Could you check a few things on this model? Use its own coordinates, in mm. Face numbers are marked on the shaded views. Coordinates: 2 decimals unless noted, no trailing zeros. Order: outer loops, then holes, each group sorted by start corner. A loop starts at its lowest first (then second) coordinate and runs counter-clockwise, first axis right, second up. Notation, with made-up numbers: (9.5, 81.25) - (18.5, 81.25) arc R19 cw to (18.5, 117.25) - close; hole circle Ø9 at (30, -0.5). An arc over 180 degrees is marked (long way). One line per item, written item: value.
from build123d import *

# Parameters (mm, degrees)
EXTRUDE_1_DEPTH     = 1.56
SKETCH_3_W          = 59.16
SKETCH_3_H          = 29.5
EXTRUDE_2_DEPTH     = 1
SKETCH_8_W          = 51
SKETCH_8_H          = 5
EXTRUDE_6_DEPTH     = 3.68
SKETCH_9_W          = 49.12
SKETCH_9_H          = 24.52
CUT_EXTRUDE_1_DEPTH = 0.1


with BuildPart() as part:
    # 草图1 → 凸台-拉伸1 (new body)
    with BuildSketch(Plane(origin=(0, 0, 0), x_dir=(1, 0, 0), z_dir=(0, 1, 0))):
        with BuildLine():
            Line((-29.5, 15.375), (29.5, 15.375))
            ThreePointArc((29.5, 15.375), (31.621320344, 14.496320344), (32.5, 12.375))
            Line((32.5, 12.375), (32.5, -12.375))
            ThreePointArc((32.5, -12.375), (31.621320344, -14.496320344), (29.5, -15.375))
            Line((29.5, -15.375), (-29.5, -15.375))
            ThreePointArc((-29.5, -15.375), (-31.621320344, -14.496320344), (-32.5, -12.375))
            Line((-32.5, -12.375), (-32.5, 12.375))
            ThreePointArc((-32.5, 12.375), (-31.621320344, 14.496320344), (-29.5, 15.375))
        make_face()
    extrude(amount=EXTRUDE_1_DEPTH)

    # 草图3 → 凸台-拉伸2 (add)
    with BuildSketch(Plane(origin=(0, 1.56, 0), x_dir=(1, 0, 0), z_dir=(0, 1, 0))):
        with Locations((0.06, -0.125)):
            Rectangle(SKETCH_3_W, SKETCH_3_H)
    extrude(amount=EXTRUDE_2_DEPTH)

    # 草图8 → 凸台-拉伸6 (add)
    with BuildSketch(Plane.XZ):
        with Locations((-0.2, -11.235)):
            Rectangle(SKETCH_8_W, SKETCH_8_H)
    extrude(amount=EXTRUDE_6_DEPTH)

    # 草图9 → 切除-拉伸1 (cut)
    with BuildSketch(Plane(origin=(0, 2.56, 0), x_dir=(1, 0, 0), z_dir=(0, 1, 0))):
        with Locations((2.45, -0.235)):
            Rectangle(SKETCH_9_W, SKETCH_9_H)
    extrude(amount=-CUT_EXTRUDE_1_DEPTH, mode=Mode.SUBTRACT)


solid = part.part
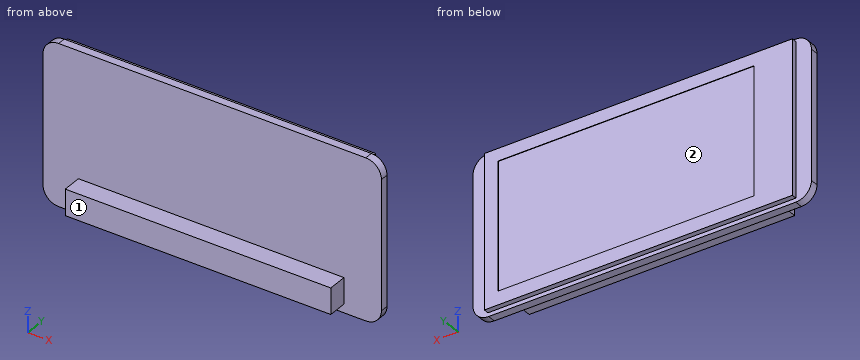
Item 1: I want a section at D-D on x = -28. Please give me the cut outline in (y, z) (3 decimals), then the cut area to 3 significant figures.
Conclusion:
outline: (0, -15.375) - (1.56, -15.375) - (1.56, -14.625) - (2.56, -14.625) - (2.56, 14.875) - (1.56, 14.875) - (1.56, 15.375) - (0, 15.375) - close
area: 77.5 mm²
Item 2: I want a section at B-B on z = 3.5. Please give me the cut outline in (x, y).
Conclusion:
outline: (-32.5, 0) - (32.5, 0) - (32.5, 1.56) - (29.64, 1.56) - (29.64, 2.56) - (27.01, 2.56) - (27.01, 2.46) - (-22.11, 2.46) - (-22.11, 2.56) - (-29.52, 2.56) - (-29.52, 1.56) - (-32.5, 1.56) - close
Item 3: I want a section at A-A on x = 19. Please give me the cut outline in (y, z) (3 decimals).
Conclusion:
outline: (-3.68, -13.735) - (0, -13.735) - (0, -15.375) - (1.56, -15.375) - (1.56, -14.625) - (2.56, -14.625) - (2.56, -12.025) - (2.46, -12.025) - (2.46, 12.495) - (2.56, 12.495) - (2.56, 14.875) - (1.56, 14.875) - (1.56, 15.375) - (0, 15.375) - (0, -8.735) - (-3.68, -8.735) - close
Item 4: Thinking about a two-plate mould opening in Z: for the marked faces 1 and 2, which applies, pulls with the +Z half, pulls with the -Z half, needs draft (parallel to the pull), parting line crosses it, or undercut?
Conclusion:
face 1: needs draft
face 2: undercut
Item 5: I want a section at C-C on y = -0.75. Please give me the cut outline in (x, z) (3 decimals).
Conclusion:
outline: (-25.7, -13.735) - (25.3, -13.735) - (25.3, -8.735) - (-25.7, -8.735) - close
Item 6: I'm going to push flat-ended pins straight in: pin 1 Ø3 at (x, y) = (-7.5, -2.5) entering from -Z (3 decimals); pin 2 Ø1.1 at (x, y) = (-5.5, 2) entering from +Z (3 decimals); pin 3 Ø3 at (y, z) = (-2.5, 0) entering from -X; pin 4 Ø12.5 at (x, z) = (2, -3.5) entering from +Y. Where does each tip first touch, or does it pass through?
Conclusion:
pin 1: z = -13.735
pin 2: z = 15.375
pin 3: through
pin 4: y = 2.46
Item 7: If I drill on probe 1 along Z at (x, y) = (-4.5, -3.25) (3 decimals); probe 2 along Y at (x, z) = (20, 1.5); probe 3 along Y at (x, z) = (-30, -12), over which ranges is the centre line in solid material (lowest first)?
Conclusion:
probe 1: -13.735 to -8.735
probe 2: 0 to 2.46
probe 3: 0 to 1.56
